Could you check a few things on this model? Use its own coordinates, in mm. Face numbers are marked on the shaded views. A direction names the side the tool comes from. Give positions to 0.01 mm unless a question says otherwise; leave off trailing zeros. Order: outer loops, then holes, each group sorted by start corner. A loop starts at its lowest first (then second) coordinate and runs counter-clockwise, first axis right, second up. Notation, with made-up numbers: (9, 70) -> (47, 70) arc R19 ccw to (47, 86) -> close; hole circle Ø11 at (-5.75, 24.5). An arc over 180 degrees is marked (long way). Write each question's results on one line, items separated by ' | '.
```python
from build123d import *

# Parameters (mm, degrees)
F0_W      = 25
F0_H      = 56
F1_DEPTH  = 25
F4_D      = 15
F5_D      = 8
F5_DEPTH  = 20
F5_TIP    = 2.4034424761
F7_DEPTH  = 1
F8_W      = 25
F8_H      = 2
F9_DEPTH  = 8
F10_W     = 1.25
F10_H     = 3
F11_DEPTH = 26.001
F12_W     = 17.5
F12_H     = 3
F13_DEPTH = 15
F14_R     = 4
F15_R     = 4
F16_DEPTH = 7
F18_D     = 9


with BuildPart() as f1:
    # F0 (on Top) → F1 (new body)
    with BuildSketch(Plane.XY):
        with Locations((12.5, 28)):
            Rectangle(F0_W, F0_H)
    extrude(amount=F1_DEPTH)

    # F4 (through all)
    with Locations(Plane.XZ):
        with Locations((12.5, 0)):
            Hole(F4_D / 2)

    # F5
    with Locations(Plane.YZ.offset(25)):
        with Locations((13, 17), (43, 17)):
            Hole(F5_D / 2, depth=F5_DEPTH)
            with Locations((0, 0, -(F5_DEPTH + F5_TIP / 2))):  # 118° drill point
                Cone(0, F5_D / 2, F5_TIP, mode=Mode.SUBTRACT)

    # F6 (on face) → F7 (join)
    with BuildSketch(Plane.XY.offset(25)):
        with BuildLine():
            ThreePointArc((12.5, 17.5), (8, 13), (12.5, 8.5))
            Line((12.5, 8.5), (12.5, 17.5))
        make_face()
        with BuildLine():
            ThreePointArc((12.5, 47.5), (8, 43), (12.5, 38.5))
            Line((12.5, 38.5), (12.5, 47.5))
        make_face()
        with BuildLine():
            Line((12.5, 47.5), (12.5, 38.5))
            ThreePointArc((12.5, 38.5), (15.6819805153, 39.8180194847), (17, 43))
            ThreePointArc((17, 43), (15.6819805153, 46.1819805153), (12.5, 47.5))
        make_face()
        with BuildLine():
            Line((12.5, 17.5), (12.5, 8.5))
            ThreePointArc((12.5, 8.5), (15.6819805153, 9.8180194847), (17, 13))
            ThreePointArc((17, 13), (15.6819805153, 16.1819805153), (12.5, 17.5))
        make_face()
    extrude(amount=F7_DEPTH)

    # F8 (on face) → F9 (join)
    with BuildSketch(Plane(origin=(0, 0, 0), x_dir=(1, 0, 0), z_dir=(0, 0, -1))):
        with Locations((12.5, -1)):
            Rectangle(F8_W, F8_H)
        with Locations((12.5, -27)):
            Rectangle(F8_W, F8_H)
        with Locations((12.5, -29)):
            Rectangle(F8_W, F8_H)
        with Locations((12.5, -55)):
            Rectangle(F8_W, F8_H)
    extrude(amount=-F9_DEPTH)

    # F10 (on face) → F11 (cut, through all)
    with BuildSketch(Plane(origin=(0, 0, 0), x_dir=(1, 0, 0), z_dir=(0, 0, -1))):
        with Locations((4.375, -6.75)):
            Rectangle(F10_W, F10_H)
        with Locations((20.625, -6.75)):
            Rectangle(F10_W, F10_H)
        with Locations((4.375, -21.25)):
            Rectangle(F10_W, F10_H)
        with Locations((20.625, -21.25)):
            Rectangle(F10_W, F10_H)
        with Locations((20.625, -49.25)):
            Rectangle(F10_W, F10_H)
        with Locations((4.375, -49.25)):
            Rectangle(F10_W, F10_H)
        with Locations((20.625, -34.75)):
            Rectangle(F10_W, F10_H)
        with Locations((4.375, -34.75)):
            Rectangle(F10_W, F10_H)
    extrude(amount=-F11_DEPTH, mode=Mode.SUBTRACT)

    # F12 (on face) → F13 (cut)
    with BuildSketch(Plane.XY.offset(25)):
        with Locations((12.5, 6.75)):
            Rectangle(F12_W, F12_H)
        with Locations((12.5, 21.25)):
            Rectangle(F12_W, F12_H)
        with Locations((12.5, 34.75)):
            Rectangle(F12_W, F12_H)
        with Locations((12.5, 49.25)):
            Rectangle(F12_W, F12_H)
    extrude(amount=-F13_DEPTH, mode=Mode.SUBTRACT)

    # F14 (on face) + F15 (on face) → F16 (join)
    with BuildSketch(Plane.XY.offset(26)):
        with Locations((12.5, 43)):
            Circle(F14_R)
    with BuildSketch(Plane.XY.offset(26)):
        with Locations((12.5, 13)):
            Circle(F15_R)
    extrude(amount=F16_DEPTH)

    # F18 (through all)
    with Locations(Plane.XZ):
        with Locations((12.5, 0)):
            Hole(F18_D / 2)


solid = f1.part
```
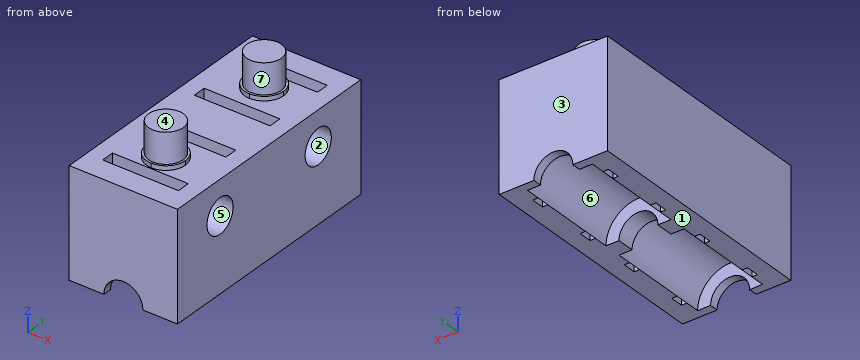
Q1. For the marked faces 5, 6 and 7, which set-ups out of +Z, -Z, +X, -X, +Y, -Y let a thin tool reach every point of the face, with its end or its side?
Here are the results:
face 5: +X | face 6: -Z | face 7: +Z
Q2. Thinking about a two-plate mould opening in Z: for the marked faces 1, 2, 3 and 4, which applies, +Z half, -Z half, draft (parallel to the pull), parting line (faces both ways), or undercut?
Here are the results:
face 1: -Z half | face 2: undercut | face 3: draft | face 4: +Z half
Q3. I need wall thicknesses on line 1 along Y through (x, z) = (21, 6.5); line 2 along X through (y, z) = (22.5, 9.5); line 3 along X through (y, z) = (21, 19). Which ranges of each line are inside material? Lowest first, please.
Here are the results:
line 1: y = 0 to 5.25, 8.25 to 19.75, 22.75 to 33.25, 36.25 to 47.75, 50.75 to 56 | line 2: x = 0 to 3.75, 5 to 20, 21.25 to 25 | line 3: x = 0 to 3.75, 21.25 to 25
Q4. Suppose I cut it at C-C on z = 28. Please give me the cut outline in (x, y).
Here are the results:
outline: circle Ø8 at (12.5, 13); circle Ø8 at (12.5, 43)
Q5. Suppose I cut it at B-B on x = 6.5. State how many separate pieces and enclosed holes the cut face has, and give its area (3 significant figures).
Here are the results:
separate pieces: 1 | enclosed holes: 2 | area: 903 mm²
Q6. Suppose I cut it at A-A on z = 22. Please give me the cut outline in (x, y), and give its area (3 significant figures).
Here are the results:
outline: (0, 0) -> (25, 0) -> (25, 56) -> (0, 56) -> close; hole (3.75, 5.25) -> (21.25, 5.25) -> (21.25, 8.25) -> (3.75, 8.25) -> close; hole (3.75, 19.75) -> (21.25, 19.75) -> (21.25, 22.75) -> (3.75, 22.75) -> close; hole (3.75, 33.25) -> (21.25, 33.25) -> (21.25, 36.25) -> (3.75, 36.25) -> close; hole (3.75, 47.75) -> (21.25, 47.75) -> (21.25, 50.75) -> (3.75, 50.75) -> close | area: 1,190 mm²
Q7. Suppose I cut it at D-D on y = 25. Please give me the cut outline in (x, z), and give its area (3 significant figures).
Here are the results:
outline: (0, 0) -> (5, 0) arc R7.5 cw to (20, 0) -> (25, 0) -> (25, 25) -> (0, 25) -> close | area: 537 mm²
Q8. I'm going to push flat-ended pins straight in: pin 1 Ø0.9 at (x, y) = (11.5, 21.5) entering from +Z; pin 2 Ø4 at (x, y) = (10, 23) entering from -Z; pin 3 Ø2 at (x, z) = (2.5, 27.5) entering from -Y. Where does each tip first touch, or does it pass through?
Here are the results:
pin 1: stops at z = 10 | pin 2: stops at z = 6 | pin 3: passes through
